The drawing under review shows one solid part. Ordinate dimensions are in mm from its lowest x, y, z. Round coordinates to 2 decimals unless told otherwise and drop trailing zeros. Loops run counter-clockwise (first coordinate to the right, second up) from the corner with the lowest first, then second, coordinate; pieces in that order, holes last. Notation, with made-up numbers: (88.25, -27.75) -> (106.25, -27.75) arc R31 cw to (106.25, 0.25) -> close; hole circle Ø2 at (14, -33). An arc over 180 degrees is marked (long way). Use a Markdown table: item, result. Add a question column.
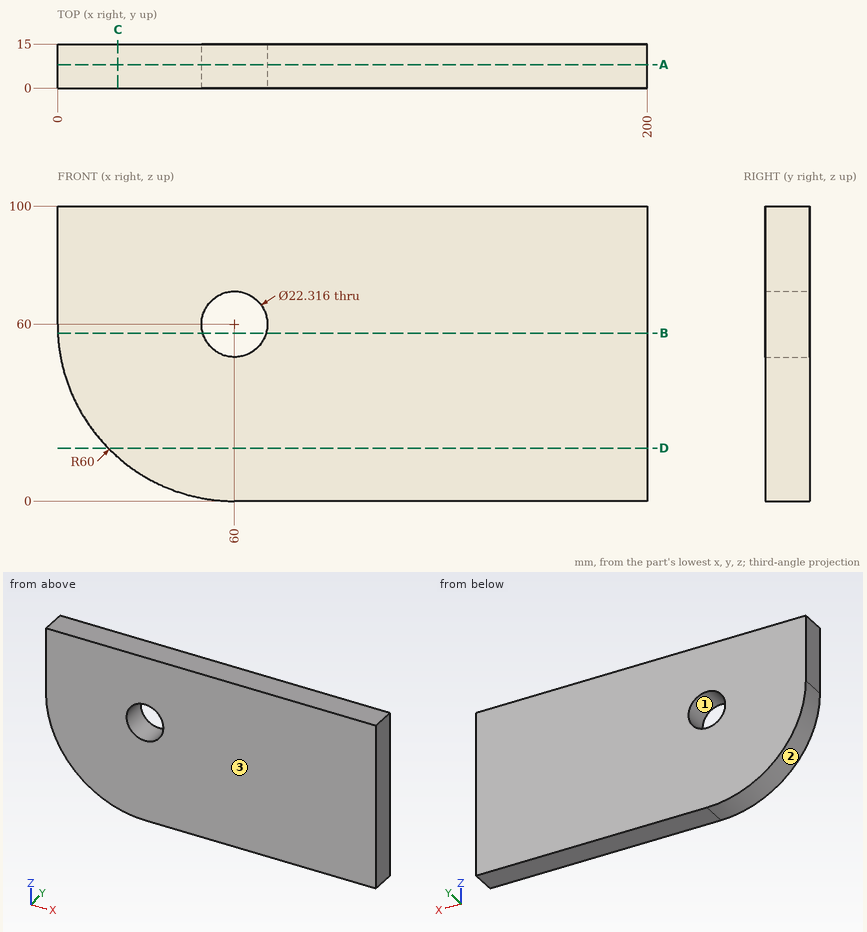
1. Consider section A-A on y = 8. State the section outline as (x, z) points, plus the area to 3 significant figures.
2. To check wall thickness, follow probe 1 along X at (y, z) = (8.5, 60); probe 2 along Z at (x, y) = (70, 1); probe 3 along X at (y, z) = (10.5, 56.5) (1 decimal). State the ranges of each line that lie inside material, in increasing order. Write a range as from..to.
3. Consider section D-D on z = 18. State the section outline as (x, y) points.
4. Consider section C-C on x = 20.5. State the section outline as (y, z) points.
5. Insertion check: P1, Ø1.5, axis at y = 5.5, z = 26.5, coming from the -X side. The pin has a flat end and moves straight along its axis. Give the tip position at first contact, or say it passes through.
6. Consider section B-B on z = 57. State the section outline as (x, y) points (3 decimals).
7. Mouldability with a two-part tool opening along X and no side actions: class the marked faces 1, 2 and 3 as +X half, -X half, draft (parallel to the pull), parting line (faces both ways), or undercut.
Verdict:
| question | item | result |
|---|---|---|
| 1 | outline | (0, 60) arc R60 ccw to (60, 0) -> (200, 0) -> (200, 100) -> (0, 100) -> close; hole circle Ø22.32 at (60, 60) |
| 1 | area | 18,800 mm² |
| 2 | probe 1 | x = 0..48.84, 71.16..200 |
| 2 | probe 2 | z = 0..55.05, 64.95..100 |
| 2 | probe 3 | x = 0.1..49.4, 70.6..200 |
| 3 | outline | (17.15, 0) -> (200, 0) -> (200, 15) -> (17.15, 15) -> close |
| 4 | outline | (0, 14.84) -> (15, 14.84) -> (15, 100) -> (0, 100) -> close |
| 5 | P1 | stops at x = 9.73 |
| 6 | outline | (0.075, 0) -> (49.253, 0) -> (49.253, 15) -> (0.075, 15) -> close; (70.747, 0) -> (200, 0) -> (200, 15) -> (70.747, 15) -> close |
| 7 | face 1 | undercut |
| 7 | face 2 | -X half |
| 7 | face 3 | draft |
